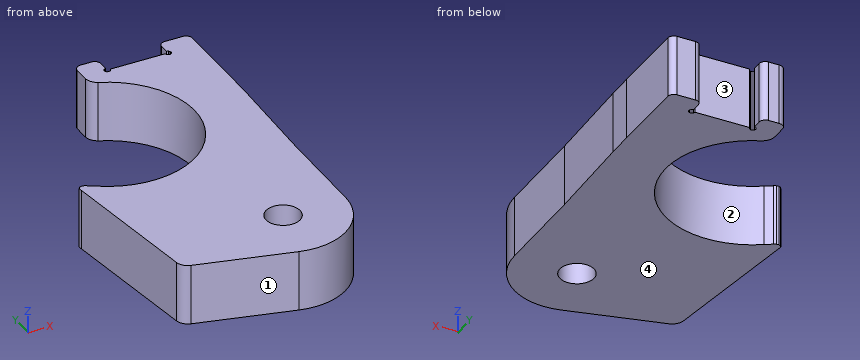
from build123d import *

# Parameters (mm, degrees)
ESQUISSE1_R        = 1.4
BOSS_EXTRU_1_DEPTH = 5


with BuildPart() as part:
    # Esquisse1 → Boss.-Extru.1 (new body)
    with BuildSketch(Plane(origin=(0, 0, 0), x_dir=(-1, 0, 0), z_dir=(0, 0, -1))):
        with BuildLine():
            Line((-15.185840881, 0.170296169), (-7.386227588, 2.157766419))
            ThreePointArc((-7.386227588, 2.157766419), (-6.883257057, 2.465245864), (-6.640893239, 3.002630961))
            Line((-6.640893239, 3.002630961), (-5.14541723, 14.953309043))
            Line((-5.14541723, 14.953309043), (-5.116713392, 15.234944478))
            Line((-5.116713392, 15.234944478), (-5.20171731, 15.387969012))
            Line((-5.20171731, 15.387969012), (-5.386870175, 15.451048966))
            Line((-5.386870175, 15.451048966), (-5.582053032, 15.438258975))
            Line((-5.582053032, 15.438258975), (-5.757396903, 15.351569039))
            Line((-5.757396903, 15.351569039), (-6.353216099, 14.974428283))
            ThreePointArc((-6.353216099, 14.974428283), (-16.665635969, 17.453925295), (-13.127159197, 27.452579762))
            ThreePointArc((-13.127159197, 27.452579762), (-12.708604135, 27.821584741), (-12.552929618, 28.357419099))
            Line((-12.552929618, 28.357419099), (-12.552929618, 29.66633814))
            ThreePointArc((-12.552929618, 29.66633814), (-12.746735333, 30.012603591), (-13.119010387, 30.149977907))
            Line((-13.119010387, 30.149977907), (-13.999989741, 30.149977907))
            ThreePointArc((-13.999989741, 30.149977907), (-14.353542873, 30.003531405), (-14.499989375, 29.649978273))
            Line((-14.499989375, 29.649978273), (-14.499989375, 28.899978823))
            Line((-14.499989375, 28.899978823), (-14.374989466, 28.866488848))
            Line((-14.374989466, 28.866488848), (-14.283479534, 28.774978915))
            Line((-14.283479534, 28.774978915), (-14.249989558, 28.649979006))
            Line((-14.249989558, 28.649979006), (-14.283479534, 28.524979098))
            Line((-14.283479534, 28.524979098), (-14.374989466, 28.433469165))
            Line((-14.374989466, 28.433469165), (-14.499989375, 28.399979189))
            Line((-14.499989375, 28.399979189), (-14.624989283, 28.433469165))
            Line((-14.624989283, 28.433469165), (-14.716499216, 28.524979098))
            Line((-14.716499216, 28.524979098), (-14.749989192, 28.649979006))
            Line((-14.749989192, 28.649979006), (-19.249985894, 28.649979006))
            Line((-19.249985894, 28.649979006), (-19.28347587, 28.524979098))
            Line((-19.28347587, 28.524979098), (-19.374985803, 28.433469165))
            Line((-19.374985803, 28.433469165), (-19.499985711, 28.399979189))
            Line((-19.499985711, 28.399979189), (-19.624985619, 28.433469165))
            Line((-19.624985619, 28.433469165), (-19.716495552, 28.524979098))
            Line((-19.716495552, 28.524979098), (-19.749985528, 28.649979006))
            Line((-19.749985528, 28.649979006), (-19.716495552, 28.774978915))
            Line((-19.716495552, 28.774978915), (-19.624985619, 28.866488848))
            Line((-19.624985619, 28.866488848), (-19.499985711, 28.899978823))
            Line((-19.499985711, 28.899978823), (-19.499985711, 29.649978273))
            ThreePointArc((-19.499985711, 29.649978273), (-19.646432213, 30.003531405), (-19.999985345, 30.149977907))
            Line((-19.999985345, 30.149977907), (-21.499984246, 30.149977907))
            ThreePointArc((-21.499984246, 30.149977907), (-21.853537377, 30.003531405), (-21.999983879, 29.649978273))
            Line((-21.999983879, 29.649978273), (-21.999983879, 23.212152991))
            Line((-21.999983879, 23.212152991), (-21.974503898, 21.118714525))
            Line((-21.974503898, 21.118714525), (-21.716894087, 13.069840423))
            Line((-21.716894087, 13.069840423), (-21.649985688, 5.150180005))
            ThreePointArc((-21.649985688, 5.150180005), (-19.62980681, 1.087138091), (-15.185840881, 0.170296169))
        make_face()
        with Locations((-16.500427031, 5.114893226)):
            Circle(ESQUISSE1_R, mode=Mode.SUBTRACT)
    extrude(amount=-BOSS_EXTRU_1_DEPTH)


solid = part.part
Part model, mm, in its own coordinate system. Face numbers are marked on the shaded views. Coordinates: 2 decimals unless noted, no trailing zeros. Loops run counter-clockwise (first coordinate to the right, second up) from the corner with the lowest first, then second, coordinate; pieces in that order, holes last. Notation, with made-up numbers: M -8.5,-11.5 L 4.5,-11.5 A14 cw 4.5,5.5 Z; hole C 44.5,65.25 d9. An arc over 180 degrees is marked long. Use a Markdown table: item, result. Add a question column.
Q1. Cut at C-C (x = 11.5). Write the cut outline in (y, z), and give its area (3 significant figures).
Q2. Probe L1, parallel to Y at x = 15.75, z = 0.7; L2, parallel to Y at x = 13.75, z = 2.85; L3, parallel to X at y = 6, z = 0.8. List the from-to ranges inside material, lowest first.
Q3. Cut at A-A (y = 4.5). Write the cut outline in (x, z).
Q4. Pin check, flat tips, straight feed: P1, Ø1, axis at y = 10.5, z = 1.5, coming from the +X side; P2, Ø1, axis at y = 4.5, z = 1.5, coming from the -X side; P3, Ø1.5, axis at y = 7, z = 3.5, coming from the -X side. Stop position of each tip, or through.
Q5. Mould opens along Y. For the marked faces 1, 2, 3 and 4 say: +Y half, -Y half, draft (parallel to the pull), parting line (faces both ways), or undercut.
Q6. Cut at B-B (x = 13.5). Write the cut outline in (y, z), and give its area (3 significant figures).
Q7. Cut at D-D (y = 28). Write the cut outline in (x, z), and give its area (3 significant figures).
Worked out:
| question | item | result |
|---|---|---|
| 1 | outline | M 1.11,0 L 13.81,0 L 13.81,5 L 1.11,5 Z |
| 1 | area | 63.5 mm2 |
| 2 | L1 | y = 0.06 to 3.93, 6.3 to 16.14, 25.58 to 28.65 |
| 2 | L2 | y = 0.54 to 14.56, 27.16 to 30.15 |
| 2 | L3 | x = 6.27 to 15.42, 17.59 to 21.66 |
| 3 | outline | M 6.45,0 L 15.24,0 L 15.24,5 L 6.45,5 Z; M 17.76,0 L 21.6,0 L 21.6,5 L 17.76,5 Z |
| 4 | P1 | stops at x = 21.7 |
| 4 | P2 | stops at x = 6.39 |
| 4 | P3 | stops at x = 6.05 |
| 5 | face 1 | -Y half |
| 5 | face 2 | undercut |
| 5 | face 3 | +Y half |
| 5 | face 4 | draft |
| 6 | outline | M 0.6,0 L 14.43,0 L 14.43,5 L 0.6,5 Z; M 27.29,0 L 30.15,0 L 30.15,5 L 27.29,5 Z |
| 6 | area | 83.5 mm2 |
| 7 | outline | M 12.62,0 L 22,0 L 22,5 L 12.62,5 Z |
| 7 | area | 46.9 mm2 |
